Build history of the part. All positions in model axes, mm. Face numbers are marked on the shaded views. A direction names the side the tool comes from. Round coordinates to 2 decimals unless told otherwise and drop trailing zeros. Order: outer loops, then holes, each group sorted by start corner. A loop starts at its lowest first (then second) coordinate and runs counter-clockwise, first axis right, second up. Notation, with made-up numbers: M -22,-30 L 3,-30 A11 ccw 3,-12 Z; hole C 31.5,67.5 d8. An arc over 180 degrees is marked long. One line per item, written item: value. Start each with the question number.
Item 1: Band-saw the part on D-D, the plane x = 12. Write the cut outline in (y, z).
Item 2: Band-saw the part on A-A, the plane z = 48. Write the cut outline in (x, y), then the cut area to 3 significant figures.
Item 3: Pin check, flat tips, straight feed: pin 1 (6 mm diameter, centred on x = 9.5, z = 8.5, fed in from +Y); pin 2 (13 mm diameter, centred on y = 15, z = 22, fed in from -X); pin 3 (9 mm diameter, centred on x = 6.5, y = 17, fed in from -Z). Stop position of each tip, or through.
Item 4: Tool access for the marked faces 1, 2 and 3: list every direction of +Z, -Z, +X, -X, +Y, -Y with a clear straight run to the whole face (end or side of a thin tool).
Item 5: Band-saw the part on B-B, the plane x = 7.5. Write the cut outline in (y, z), then the cut area to 3 significant figures.
Item 6: Band-saw the part on C-C, the plane y = 8.25. Write the cut outline in (x, z), then the cut area to 3 significant figures.
Item 7: Probe L1, parallel to Z at x = 12.25, y = 15; L2, parallel to Z at x = 9.25, y = 5.5; L3, parallel to Z at x = 7.5, y = 6. List the from-to ranges inside material, lowest first.
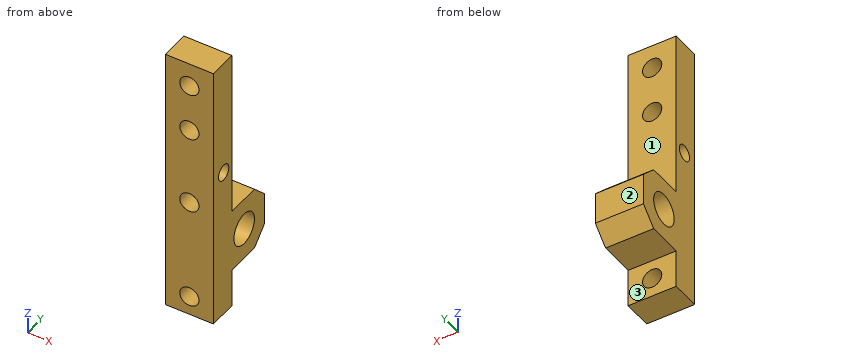
```python
from build123d import *

# Parameters (mm, degrees)
F0_R     = 5
F0_R_2   = 2.5
F1_DEPTH = 15
F2_SIZE  = 5
F3_R     = 3
F4_DEPTH = 9


with BuildPart() as f1:
    # F0 (on Right) → F1 (new body)
    with BuildSketch(Plane.YZ):
        Polygon((0, 85), (0, 0), (9, 0), (9, 12), (25, 12), (25, 32), (9, 32), (9, 85), align=None)
        with Locations((15, 22)):
            Circle(F0_R, mode=Mode.SUBTRACT)
        with Locations((5, 48)):
            Circle(F0_R_2, mode=Mode.SUBTRACT)
    extrude(amount=F1_DEPTH)

    # F2
    f2_edges = [f1.edges().sort_by_distance(p)[0] for p in [
        (7.5, 25, 32),
        (7.5, 25, 12),
    ]]
    chamfer(f2_edges, length=F2_SIZE)

    # F3 (on face) → F4 (cut, through all)
    with BuildSketch(Plane(origin=(0, 9, 0), x_dir=(-1, 0, 0), z_dir=(0, 1, 0))):
        with Locations((-7.5, 77.5)):
            Circle(F3_R)
        with Locations((-7.5, 62.5)):
            Circle(F3_R)
        with Locations((-7.5, 6)):
            Circle(F3_R)
        with Locations((-7.5, 38)):
            Circle(F3_R)
    extrude(amount=-F4_DEPTH, mode=Mode.SUBTRACT)


solid = f1.part
```
Output:
1. outline: M 0,0 L 9,0 L 9,12 L 20,12 L 25,17 L 25,27 L 20,32 L 9,32 L 9,85 L 0,85 Z; hole C 5,48 d5; hole C 15,22 d10
2. outline: M 0,0 L 15,0 L 15,2.5 L 0,2.5 Z; M 0,7.5 L 15,7.5 L 15,9 L 0,9 Z
2. area: 60.0 mm²
3. pin 1: stops at y = 9
3. pin 2: stops at x = 0
3. pin 3: stops at z = 12
4. face 1: +Z, +X, -X, +Y
4. face 2: +Z, -Z, +X, -X, +Y
4. face 3: -Z, +X, -X, +Y
5. outline: M 0,0 L 9,0 L 9,3 L 0,3 Z; M 0,9 L 9,9 L 9,12 L 20,12 L 25,17 L 25,27 L 20,32 L 9,32 L 9,35 L 0,35 Z; M 0,41 L 9,41 L 9,59.5 L 0,59.5 Z; M 0,65.5 L 9,65.5 L 9,74.5 L 0,74.5 Z; M 0,80.5 L 9,80.5 L 9,85 L 0,85 Z; hole C 5,48 d5; hole C 15,22 d10
5. area: 746 mm²
6. outline: M 0,0 L 15,0 L 15,85 L 0,85 Z; hole C 7.5,6 d6; hole C 7.5,38 d6; hole C 7.5,62.5 d6; hole C 7.5,77.5 d6
6. area: 1,160 mm²
7. L1: z = 12 to 17, 27 to 32
7. L2: z = 0 to 3.56, 8.44 to 35.56, 40.44 to 45.55, 50.45 to 60.06, 64.94 to 75.06, 79.94 to 85
7. L3: z = 0 to 3, 9 to 35, 41 to 45.71, 50.29 to 59.5, 65.5 to 74.5, 80.5 to 85
